```python
from build123d import *

# Parameters (mm, degrees)
F0_W     = 5
F0_H     = 15
F1_DEPTH = 5
F2_W     = 10
F2_H     = 5
F3_DEPTH = 5
F6_R     = 5


with BuildPart() as f1:
    # F0 (on Front) → F1 (new body)
    with BuildSketch(Plane.XZ):
        with Locations((0, 122.5)):
            Rectangle(F0_W, F0_H)
    extrude(amount=F1_DEPTH)

    # F2 (on Front) → F3 (join)
    with BuildSketch(Plane.XZ):
        with Locations((0, 125)):
            Rectangle(F2_W, F2_H)
    extrude(amount=F3_DEPTH)

    # F4 (on Front) → F5 (revolve)
    with BuildSketch(Plane.XZ):
        with BuildLine():
            Line((0, 0), (0, 116.0027790625))
            ThreePointArc((0, 116.0027790625), (-11.5318288714, 106.5712142822), (-4.5754415185, 93.3975220769))
            Line((-4.5754415185, 93.3975220769), (-22.5224215537, 73.0274617672))
            Line((-22.5224215537, 73.0274617672), (-4.5754415185, 57.2153292803))
            add(Edge.make_bspline(
                [(-4.5754415185, 57.2153292803), (-4.4751641327, 56.0238017391), (-4.1175165379, 51.7741201604), (-8.9838991311, 12.8241412869), (-19.6573992459, 13.3243982282), (-23.4876684844, 13.5039193556)],
                knots=[0, 0, 0, 0, 0.1998744201, 0.7128686595, 1, 1, 1, 1], degree=3))
            Line((-23.4876684844, 13.5039193556), (-23.4876684844, 0))
            Line((-23.4876684844, 0), (0, 0))
        make_face()
    revolve(axis=Axis((0, 0, 58.0013895312), (0, 0, 1)))

    # F6
    f6_edges = [f1.edges().sort_by_distance(p)[0] for p in [
        (22.522422, 0, 73.027462),
    ]]
    fillet(f6_edges, radius=F6_R)


solid = f1.part
```
Design review of the part built by this model. Coordinates are the model's own, in mm. A direction names the side the tool comes from. Round coordinates to 2 decimals unless told otherwise and drop trailing zeros. Write each loop counter-clockwise with the first axis right and the second up, starting at its lowest first coordinate (ties: lowest second). Pieces come first, ordered by that corner, then holes. Notation, with made-up numbers: (29.5, -0.75) -> (86.5, -0.75) arc R19 ccw to (86.5, 3.25) -> close; hole circle Ø1 at (35.25, 87.5). An arc over 180 degrees is marked (long way). Write item = value, one per line. Start each with the question number.
1) Tool access review of faces 1 (the face through (4, -2, 122.5)), 2 (the face through (-2.5, -2, 129)), 3 (the face through (-6.79, -2.14, 90.51)), 4 (the face through (0, -5, 123)), 5 (the face through (4, -2, 127.5)): name each direction out of +Z, -Z, +X, -X, +Y, -Y from which nothing blocks a thin tool from reaching the whole face with its end or side.
2) Take a section at B-B, the plane y = -7. Count the separate pieces of the cut face and the enclosed holes in it, plus the area to 3 significant figures.
3) Take a section at C-C, the plane z = 90.5. State the section outline as (x, y) points, plus the area to 3 significant figures.
4) Take a section at A-A, the plane z = 9.5. State the section outline as (x, y) points.
5) Clearance check with flat-ended pins moving along their axes: pin 1 (0.8 mm diameter, centred on y = -3, z = 128.5, fed in from +X); pin 2 (3 mm diameter, centred on y = -1.5, z = 128, fed in from -X); pin 3 (11 mm diameter, centred on x = -0.5, z = 123.5, fed in from +Y). State where each tip first meets the part, or that it passes through.
6) Mouldability with a two-part tool opening along Z and no side actions: class faces 6 (the face through (0, 0, 0)), 7 (the face through (-5, -2, 125)), 8 (the face through (-4, -2, 122.5)) as +Z half, -Z half, draft (parallel to the pull), parting line (faces both ways), or undercut.
7) Wall thickness on probe 1 along Z at (x, y) = (-19.5, -12); probe 2 along Z at (x, y) = (-15, 2.5); probe 3 along Z at (x, y) = (6, 13.5): over which ranges is each line inside the solid? List them lowest first. Write a range as from..to.
Results list:
q1.face_1 = +X, +Y, -Y
q1.face_2 = +Z, -X, +Y, -Y
q1.face_3 = none
q1.face_4 = +Z, +X, -X, -Y
q1.face_5 = +Z, +X, +Y, -Y
q2.separate_pieces = 3
q2.enclosed_holes = 0
q2.area = 1,950 mm²
q3.outline = circle Ø14.26 at (0, 0)
q3.area = 160 mm²
q4.outline = circle Ø46.98 at (0, 0)
q5.pin_1 = 2.5
q5.pin_2 = -5
q5.pin_3 = 0
q6.face_6 = -Z half
q6.face_7 = draft
q6.face_8 = undercut
q7.probe_1 = 0..13.48
q7.probe_2 = 0..14.84, 66.58..81.33
q7.probe_3 = 0..15.14, 66.2..81.82
